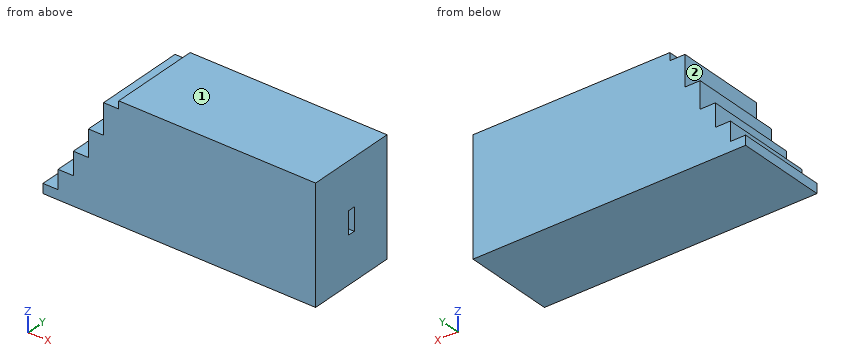
from build123d import *

# Parameters (mm, degrees)
F1_DEPTH = 152.4
F3_DEPTH = 25.4


with BuildPart() as f1:
    # F0 (on Front) → F1 (new body)
    with BuildSketch(Plane.XZ):
        Polygon((228.6, -96.8375), (228.6, 96.8375), (-101.6, 96.8375), (-101.6, 84.1375), (-127, 84.1375), (-127, 33.3375), (-152.4, 33.3375), (-152.4, -11.1125), (-177.8, -11.1125), (-177.8, -49.2125), (-203.2, -49.2125), (-203.2, -80.9625), (-228.6, -80.9625), (-228.6, -96.8375), align=None)
    extrude(amount=F1_DEPTH)

    # F2 (on face) → F3 (cut)
    with BuildSketch(Plane.YZ.offset(228.6)):
        Polygon((-82.55, 19.05), (-82.55, 8.069792), (-76.2, 0), (-69.85, 8.069792), (-69.85, 19.05), align=None)
        Polygon((-76.2, 0), (-82.55, 8.069792), (-82.55, -8.069792), align=None)
        Polygon((-69.85, 8.069792), (-76.2, 0), (-69.85, -8.069792), align=None)
        Polygon((-69.85, -8.069792), (-76.2, 0), (-82.55, -8.069792), (-82.55, -19.05), (-69.85, -19.05), align=None)
    extrude(amount=-F3_DEPTH, mode=Mode.SUBTRACT)


solid = f1.part
Could you check a few things on this model? Use its own coordinates, in mm. Face numbers are marked on the shaded views. A direction names the side the tool comes from. Coordinates: 2 decimals unless noted, no trailing zeros. Write each loop counter-clockwise with the first axis right and the second up, starting at its lowest first coordinate (ties: lowest second). Pieces come first, ordered by that corner, then holes. Notation, with made-up numbers: M 2,-17 L 6,-17 A31 ccw 6,8 Z; hole C 4,8 d8. An arc over 180 degrees is marked long. One line per question, with ' | ' between items.
1) For the marked faces 1 and 2, which set-ups out of +Z, -Z, +X, -X, +Y, -Y let a thin tool reach every point of the face, with its end or its side?
Checks:
face 1: +Z, +X, -X, +Y, -Y | face 2: +Z, -X, +Y, -Y
2) Imagine slicing it at A-A, the plane y = -33. Write out the boundary of the cut face in (x, z), and give its area (3 significant figures).
Checks:
outline: M -228.6,-96.84 L 228.6,-96.84 L 228.6,96.84 L -101.6,96.84 L -101.6,84.14 L -127,84.14 L -127,33.34 L -152.4,33.34 L -152.4,-11.11 L -177.8,-11.11 L -177.8,-49.21 L -203.2,-49.21 L -203.2,-80.96 L -228.6,-80.96 Z | area: 75,600 mm²
3) I need wall thicknesses on probe 1 along X at (y, z) = (-114, 65); probe 2 along Z at (x, y) = (-196, -145); probe 3 along X at (y, z) = (-122, -10.5). Which ranges of each line are inside material? Lowest first, please. Write a range as [from, to].
Checks:
probe 1: [-127, 228.6] | probe 2: [-96.84, -49.21] | probe 3: [-152.4, 228.6]
4) Imagine slicing it at C-C, the plane x = -116.5. Write out the boundary of the cut face in (y, z).
Checks:
outline: M -152.4,-96.84 L 0,-96.84 L 0,84.14 L -152.4,84.14 Z
5) Imagine slicing it at B-B, the plane x = -184. Write out the boundary of the cut face in (y, z).
Checks:
outline: M -152.4,-96.84 L 0,-96.84 L 0,-49.21 L -152.4,-49.21 Z
6) For pin 1 Ø12 at (x, y) = (-149.5, -64) entering from +Z; pin 2 Ø10 at (y, z) = (-46.5, 89.5) entering from -X; pin 3 Ø5 at (y, z) = (-57.5, 74) entering from -X, each with a flat end and sliding along its axis, tell me the tip position at first contact or that it passes through.
Checks:
pin 1: z = 33.34 | pin 2: x = -101.6 | pin 3: x = -127
